Can you work these out from the drawing? Everything is in mm from the part's minimum corner. A direction names the side the tool comes from. Round coordinates to 2 decimals unless told otherwise and drop trailing zeros. Write each loop counter-clockwise with the first axis right and the second up, starting at its lowest first coordinate (ties: lowest second). Pieces come first, ordered by that corner, then holes. Notation, with made-up numbers: (-26, 22) - (-15, 22) arc R5 cw to (-15, 31) - close; hole circle Ø4 at (49.25, 21.5). An arc over 180 degrees is marked (long way). Write each question's results on one line, items separated by ' | '. Start each with the question number.
(1) Imagine slicing it at A-A on x = 7.75. Write out the boundary of the cut face in (y, z), then the cut area to 3 significant figures.
(2) For P1, Ø3, axis at x = 8, y = 36, coming from the +Z side; P2, Ø4.5, axis at y = 21, z = 2, coming from the +X side; P3, Ø4.5, axis at y = 37.5, z = 2, coming from the -X side, each with a flat end and sliding along its axis, tell me the tip position at first contact or that it passes through.
(3) Please list where these lines run through material, in increasing order: line 1 (Y direction, x = 8.5, z = 2.75); line 2 (Z direction, x = 7, y = 26); line 3 (X direction, y = 5.5, z = 3.5). Write a range as [from, to].
(4) Thinking about a two-plate mould opening in Y: for the marked faces 5, 6, 7 and 8, which applies, +Y half, -Y half, draft (parallel to the pull), parting line (faces both ways), or undercut?
(5) Imagine slicing it at D-D on z = 7.5. Write out the boundary of the cut face in (x, y).
(6) Imagine slicing it at B-B on z = 2.25. Write out the boundary of the cut face in (x, y), then the cut area to 3 significant figures.
(7) Imagine slicing it at C-C on y = 7. Write out the boundary of the cut face in (x, z).
(8) On a 3-axis mill with a long thin cutter (end or side, diameter ignored), from which of +Z, -Z, +X, -X, +Y, -Y can I reach the whole of each face in a straight line? I mean the marked faces 1, 2, 3 and 4. Say none if no direction works.
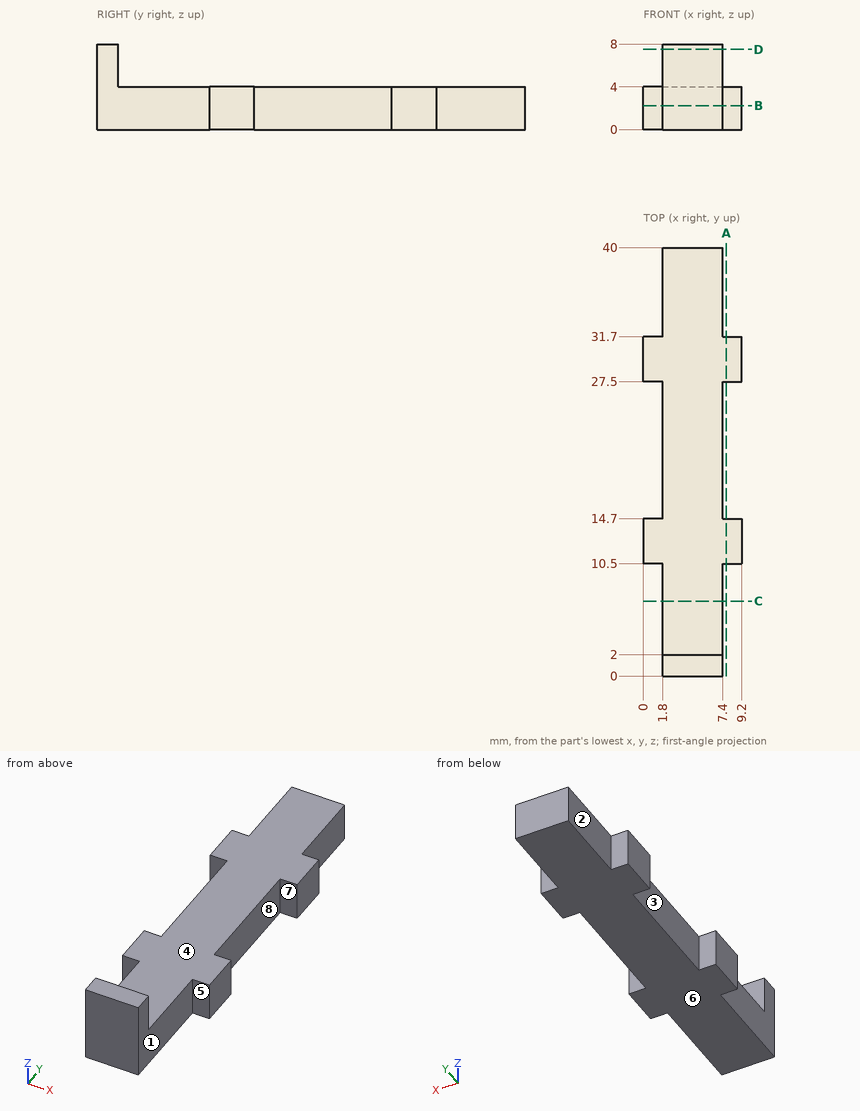
Response:
1) outline: (10.5, 0) - (14.7, 0) - (14.7, 4) - (10.5, 4) - close; (27.5, 0) - (31.7, 0) - (31.7, 4) - (27.5, 4) - close | area: 33.6 mm²
2) P1: z = 4 | P2: x = 7.4 | P3: x = 1.8
3) line 1: [10.5, 14.7], [27.5, 31.7] | line 2: [0, 4] | line 3: [1.8, 7.4]
4) face 5: -Y half | face 6: draft | face 7: undercut | face 8: undercut
5) outline: (1.8, 0) - (7.4, 0) - (7.4, 2) - (1.8, 2) - close
6) outline: (0, 10.5) - (1.8, 10.5) - (1.8, 0) - (7.4, 0) - (7.4, 10.5) - (9.2, 10.5) - (9.2, 14.7) - (7.4, 14.7) - (7.4, 27.5) - (9.2, 27.5) - (9.2, 31.7) - (7.4, 31.7) - (7.4, 40) - (1.8, 40) - (1.8, 31.7) - (0, 31.7) - (0, 27.5) - (1.8, 27.5) - (1.8, 14.7) - (0, 14.7) - close | area: 254 mm²
7) outline: (1.8, 0) - (7.4, 0) - (7.4, 4) - (1.8, 4) - close
8) face 1: +Z, -Z, +X, -Y | face 2: +Z, -Z, -X, +Y | face 3: +Z, -Z, -X | face 4: +Z, +X, -X, +Y
